Source: CAD feature listing. Evaluate the final solid. Frame: model axes, mm. A direction names the side the tool comes from. Give positions to 0.01 mm unless a question says otherwise; leave off trailing zeros. Order: outer loops, then holes, each group sorted by start corner. A loop starts at its lowest first (then second) coordinate and runs counter-clockwise, first axis right, second up. Notation, with made-up numbers: (-35.5, 41.5) - (-4.5, 41.5) arc R7 ccw to (-4.5, 48.5) - close; hole circle Ø5 at (64, 45). An arc over 180 degrees is marked (long way). Answer as CSV lines item,"result".
```python
from build123d import *

# Parameters (mm, degrees)
EXTRUDE_2_DEPTH          = 30
SKETCH_3_R               = 10.5
CUT_EXTRUDE_1_DEPTH      = 30
CUT_EXTRUDE_START        = -30
SKETCH_4_R               = 10.5
CUT_EXTRUDE_2_DEPTH      = 30
SKETCH_5_R               = 10.5
CUT_EXTRUDE_3_DEPTH      = 30
SKETCH_6_R               = 10.5
CUT_EXTRUDE_4_DEPTH      = 30
CUT_EXTRUDE_5_DEPTH      = 99.994949366
CUT_EXTRUDE_5_DEPTH_BACK = 99.994949366


with BuildPart() as part:
    # Эскиз2 → Бобышка-Вытянуть2 (new body)
    with BuildSketch(Plane(origin=(0, 0, 0), x_dir=(1, 0, 0), z_dir=(0, 1, 0))):
        Polygon((-20, 50), (-50, 50), (-50, 20), (-20, 20), (-10, 5), (-10, -5), (-20, -20), (-50, -20), (-50, -50), (-20, -50), (-5, -30), (5, -30), (20, -50), (50, -50), (50, -20), (20, -20), (10, -5), (10, 5), (20, 20), (50, 20), (50, 50), (20, 50), (5, 30), (-5, 30), align=None)
    extrude(amount=EXTRUDE_2_DEPTH)

    # Эскиз3 → Вырез-Вытянуть1 (cut)
    with BuildSketch(Plane.XY.offset(50)):
        with Locations((-35, 15)):
            Circle(SKETCH_3_R)
    extrude(amount=-CUT_EXTRUDE_1_DEPTH, mode=Mode.SUBTRACT)

    # Эскиз4 → Вырез-Вытянуть2 (cut)
    with BuildSketch(Plane(origin=(0, 0, -50), x_dir=(-1, 0, 0), z_dir=(0, 0, -1)).offset(CUT_EXTRUDE_START)):
        with Locations(Location((35, 15, 0), (0, 0, 180))):
            Circle(SKETCH_4_R)
    extrude(amount=CUT_EXTRUDE_2_DEPTH, mode=Mode.SUBTRACT)

    # Эскиз5 → Вырез-Вытянуть3 (cut)
    with BuildSketch(Plane(origin=(0, 0, -50), x_dir=(-1, 0, 0), z_dir=(0, 0, -1))):
        with Locations((-35, 15)):
            Circle(SKETCH_5_R)
    extrude(amount=-CUT_EXTRUDE_3_DEPTH, mode=Mode.SUBTRACT)

    # Эскиз6 → Вырез-Вытянуть4 (cut)
    with BuildSketch(Plane.XY.offset(50).offset(CUT_EXTRUDE_START)):
        with Locations(Location((35, 15, 0), (0, 0, 180))):
            Circle(SKETCH_6_R)
    extrude(amount=CUT_EXTRUDE_4_DEPTH, mode=Mode.SUBTRACT)

    # Эскиз7 → Вырез-Вытянуть5 (cut, two sides: drawn at the far end of the back side and taken through both)
    with BuildSketch(Plane.XY.offset(30).offset(-CUT_EXTRUDE_5_DEPTH_BACK)):
        Polygon((-20, 0), (-5, 15), (5, 15), (20, 0), align=None)
    extrude(amount=CUT_EXTRUDE_5_DEPTH + CUT_EXTRUDE_5_DEPTH_BACK, mode=Mode.SUBTRACT)


solid = part.part
```
(1) Cut plane A-A (z = 39.5). Return loops of the section in (x, y) (3 decimals).
Completed:
outline,"(-50, 0) - (-20, 0) - (-12.125, 7.875) - (-12.125, 30) - (-50, 30) - close; (12.125, 7.875) - (20, 0) - (50, 0) - (50, 30) - (12.125, 30) - close; hole circle Ø21 at (-35, 15); hole circle Ø21 at (35, 15)"
(2) Access query for faces 1 (the flat face through (0, 22, -30)), 2 (the flat face through (-12.605, 18.123, 40.14)), 3 (the flat face through (-31, 5, 20)). Directions: +Z, -Z, +X, -X, +Y, -Y. A direction counts if a zero-diameter tool reaches every point of the face in a straight line with its end or side. Return the directions, or none.
Completed:
face 1,"-Z, +Y, -Y"
face 2,"+Z, +Y, -Y"
face 3,"-X, +Y, -Y"
(3) Contact query for flat-ended pins moving along their axis: pin 1 (2 mm diameter, centred on x = -17.5, y = 22, fed in from +Z); pin 2 (8 mm diameter, centred on y = 24.5, z = -2.5, fed in from -X); pin 3 (6 mm diameter, centred on y = 15, z = -15.5, fed in from -X). Output: stop coordinate, or through.
Completed:
pin 1,"z = 48"
pin 2,"x = -11"
pin 3,"x = -19"
(4) Ray query, line 1 (Z direction, x = -22, y = 5.5); line 2 (X direction, y = 12.5, z = -39); line 3 (Y direction, x = -35, z = 36.5). Return the intervals inside material, ascending. Write a range as from..to.
Completed:
line 1,"-50..-20, 20..50"
line 2,"-50..-45.2, -24.8..-11.75, 11.75..24.8, 45.2..50"
line 3,"0..4.5, 25.5..30"
(5) Mould query, pull axis Y, two halves, no side actions, for faces 4 (the flat face through (9, 11, -1)), 5 (the cylindrical face through (-45.49, 15.46, 35.21)), 6 (the flat face through (31, 5, -20)). Classes: released by +Y, released by -Y, zero draft, split by the parting line, or undercut.
Completed:
face 4,"released by -Y"
face 5,"undercut"
face 6,"zero draft"
(6) Cut plane C-C (z = -26). Return loops of the section in (x, y).
Completed:
outline,"(-50, 0) - (-20, 0) - (-5, 15) - (5, 15) - (20, 0) - (50, 0) - (50, 30) - (-50, 30) - close; hole circle Ø21 at (-35, 15); hole circle Ø21 at (35, 15)"
(7) Cut plane D-D (y = 28.25). Return loops of the section in (x, z).
Completed:
outline,"(-50, -50) - (-20, -50) - (-5, -30) - (5, -30) - (20, -50) - (50, -50) - (50, -20) - (20, -20) - (10, -5) - (10, 5) - (20, 20) - (50, 20) - (50, 50) - (20, 50) - (5, 30) - (-5, 30) - (-20, 50) - (-50, 50) - (-50, 20) - (-20, 20) - (-10, 5) - (-10, -5) - (-20, -20) - (-50, -20) - close"
(8) Cut plane B-B (x = 35). Return loops of the section in (y, z).
Completed:
outline,"(0, -50) - (4.5, -50) - (4.5, -20) - (0, -20) - close; (0, 20) - (4.5, 20) - (4.5, 50) - (0, 50) - close; (25.5, -50) - (30, -50) - (30, -20) - (25.5, -20) - close; (25.5, 20) - (30, 20) - (30, 50) - (25.5, 50) - close"
